Source: CAD feature listing. Evaluate the final solid. Frame: model axes, mm. A direction names the side the tool comes from. Coordinates: 2 decimals unless noted, no trailing zeros. Order: outer loops, then holes, each group sorted by start corner. A loop starts at its lowest first (then second) coordinate and runs counter-clockwise, first axis right, second up.
```python
from build123d import *

# Parameters (mm, degrees)
BOSS_EXTRUDE1_DEPTH = 33.02
FILLET1_R           = 2.54
SKETCH4_R           = 9.525
CUT_EXTRUDE1_DEPTH  = 141.448449618
SKETCH5_R           = 3.175
CUT_EXTRUDE2_DEPTH  = 145.785570068
SKETCH6_W           = 14.1732
SKETCH6_H           = 19.05
CUT_EXTRUDE3_DEPTH  = 141.448449618
SKETCH7_R           = 4.826
CUT_EXTRUDE4_DEPTH  = 6.35
SKETCH8_R           = 4.826
CUT_EXTRUDE5_DEPTH  = 145.785570068
FILLET2_R           = 2.54
FILLET3_R           = 2.54


with BuildPart() as part:
    # Sketch1 → Boss-Extrude1 (new body)
    with BuildSketch(Plane.XY):
        Polygon((0, 0), (-45.72, 0), (-45.72, -133.35), (-29.21, -133.35), (-29.21, -16.51), (0, -16.51), align=None)
    extrude(amount=BOSS_EXTRUDE1_DEPTH)

    # Fillet1
    fillet1_edges = [part.edges().sort_by_distance(p)[0] for p in [
        (-45.72, 0, 16.51),
        (0, 0, 16.51),
        (-22.86, 0, 33.02),
        (-22.86, 0, 0),
    ]]
    fillet(fillet1_edges, radius=FILLET1_R)

    # Sketch4 → Cut-Extrude1 (cut, through all)
    with BuildSketch(Plane(origin=(-29.21, 0, 0), x_dir=(0, 0, -1), z_dir=(1, 0, 0))):
        with Locations(Location((-16.51, -66.548, 0), (0, 0, 90))):
            Circle(SKETCH4_R)
    extrude(amount=-CUT_EXTRUDE1_DEPTH, mode=Mode.SUBTRACT)

    # Sketch5 → Cut-Extrude2 (cut, through all)
    with BuildSketch(Plane.XY.offset(33.02)):
        with Locations((-37.465, -35.56)):
            Circle(SKETCH5_R)
        with Locations((-37.465, -99.06)):
            Circle(SKETCH5_R)
    extrude(amount=-CUT_EXTRUDE2_DEPTH, mode=Mode.SUBTRACT)

    # Sketch6 → Cut-Extrude3 (cut, through all)
    with BuildSketch(Plane(origin=(-29.21, 0, 0), x_dir=(0, 0, -1), z_dir=(1, 0, 0))):
        with Locations((-16.51, -117.475)):
            Rectangle(SKETCH6_W, SKETCH6_H)
    extrude(amount=-CUT_EXTRUDE3_DEPTH, mode=Mode.SUBTRACT)

    # Sketch7 → Cut-Extrude4 (cut)
    with BuildSketch(Plane.XZ.offset(133.35)):
        with Locations(Location((-37.465, 16.51, 0), (0, 0, 270))):
            Circle(SKETCH7_R)
    extrude(amount=-CUT_EXTRUDE4_DEPTH, mode=Mode.SUBTRACT)

    # Sketch8 → Cut-Extrude5 (cut, through all)
    with BuildSketch(Plane(origin=(0, 0, 0), x_dir=(1, 0, 0), z_dir=(0, 1, 0))):
        with Locations(Location((-11.43, -16.51, 0), (0, 0, 180))):
            Circle(SKETCH8_R)
    extrude(amount=-CUT_EXTRUDE5_DEPTH, mode=Mode.SUBTRACT)

    # Fillet2
    fillet2_edges = [part.edges().sort_by_distance(p)[0] for p in [
        (-29.21, -133.35, 16.51),
        (-45.72, -133.35, 16.51),
        (-37.465, -133.35, 33.02),
        (-37.465, -133.35, 0),
    ]]
    fillet(fillet2_edges, radius=FILLET2_R)

    # Fillet3
    fillet3_edges = [part.edges().sort_by_distance(p)[0] for p in [
        (-29.21, -16.51, 16.51),
    ]]
    fillet(fillet3_edges, radius=FILLET3_R)


solid = part.part
```
Q1. Material intervals for line 1 along X through (y, z) = (-129, 16); line 2 along Y through (x, z) = (-36, 23); line 3 along X through (y, z) = (-12, 16), sorted ascending.
Solutions:
line 1: x = -45.72 to -42.26, -32.67 to -29.21
line 2: y = -133.35 to -127, -107.95 to -101.88, -96.24 to -73.52, -59.58 to -38.38, -32.74 to 0
line 3: x = -45.72 to -16.23, -6.63 to 0
Q2. Pin query (flat end, axial travel): P1, Ø10, axis at y = -64.5, z = 12, coming from the +X side; P2, Ø5, axis at x = -37.465, y = -35.56, coming from the -Z side; P3, Ø2, axis at x = -25.5, z = 29, coming from the -Y side. Return the tip coordinate at first contact, or that it passes through.
Solutions:
P1: stops at x = -29.21
P2: passes through
P3: stops at y = -16.51
Q3. Set-up query: faces 5 (the cylindrical face through (-37.349, -132.586, 0.724)), 6 (the flat face through (-16.5, -16.51, 16.3)), 7 (the flat face through (-37, -118, 9.423)). Return all of +Z, -Z, +X, -X, +Y, -Y with unobstructed straight access to the full face (end or side cutting, diameter ignored); none if empty.
Solutions:
face 5: -Z, +X, -X, -Y
face 6: +Z, -Z, +X, -Y
face 7: +X, -X
Q4. Section query B-B on x = -11.43. Output: boundary loops of the cut face in (y, z).
Solutions:
outline: (-16.51, 0) - (-2.54, 0) arc R2.54 ccw to (0, 2.54) - (0, 11.68) - (-16.51, 11.68) - close; (-16.51, 21.34) - (0, 21.34) - (0, 30.48) arc R2.54 ccw to (-2.54, 33.02) - (-16.51, 33.02) - close
Q5. Section query D-D on x = -23. Output: boundary loops of the cut face in (y, z).
Solutions:
outline: (-16.51, 0) - (-2.54, 0) arc R2.54 ccw to (0, 2.54) - (0, 30.48) arc R2.54 ccw to (-2.54, 33.02) - (-16.51, 33.02) - close
Q6. Pull-direction query (Y, two-part tool) for faces 1 (the cylindrical face through (-28.486, -17.274, 16.741)), 2 (the flat face through (-33.7, -127, 19.8)), 3 (the cylindrical face through (-0.764, -0.724, 16.741)), 4 (the cylindrical face through (-34.203, -130.219, 20.067)); classes: pulls with the +Y half, pulls with the -Y half, needs draft (parallel to the pull), parting line crosses it, or undercut.
Solutions:
face 1: pulls with the -Y half
face 2: undercut
face 3: pulls with the +Y half
face 4: needs draft
Q7. Section query C-C on y = -99.06. Output: boundary loops of the cut face in (x, z).
Solutions:
outline: (-45.72, 0) - (-40.64, 0) - (-40.64, 33.02) - (-45.72, 33.02) - close; (-34.29, 0) - (-29.21, 0) - (-29.21, 33.02) - (-34.29, 33.02) - close
Q8. Section query A-A on z = 16.51. Give the number of separate pieces and of enclosed holes in the cut face, plus the area to 3 significant figures.
Solutions:
separate pieces: 5
enclosed holes: 2
area: 1,770 mm2
